Could you check a few things on this model? Use its own coordinates, in mm. Give positions to 0.01 mm unless a question says otherwise; leave off trailing zeros. Loops run counter-clockwise (first coordinate to the right, second up) from the corner with the lowest first, then second, coordinate; pieces in that order, holes last. Notation, with made-up numbers: (-28, -38) - (-15, -38) arc R28 cw to (-15, -1) - close; hole circle Ø3 at (-38, -2.5). An arc over 180 degrees is marked (long way). Write each question's results on one line, items separated by ' | '. Start each with the question number.
1) I want a section at C-C, the plane z = -159.5. Write out the boundary of the cut face in (x, y) (3 decimals).
2) I want a section at A-A, the plane y = -56. Write out the boundary of the cut face in (x, z).
3) If I drill on probe 1 along Z at (x, y) = (187, 12) (3 decimals); probe 2 along Z at (x, y) = (210, -17) (3 decimals); probe 3 along Y at (x, z) = (238, -112), over which ranges is the centre line in solid material (lowest first)? Write a range as [from, to].
4) I'm going to push flat-ended pins straight in: pin 1 (8 mm diameter, centred on x = 149.5, y = -143, fed in from -Z); pin 2 (15 mm diameter, centred on x = -2.5, z = 34.5, fed in from +Y); pin 3 (8 mm diameter, centred on x = 209.5, y = -24, fed in from +Z) (3 decimals). Where does each tip first touch, or does it pass through?
5) I want a section at B-B, the plane y = 7.5. Write out the boundary of the cut face in (x, z) (3 decimals).
6) I want a section at D-D, the plane x = 194. Count the separate pieces of the cut face and the enclosed holes in it, and give its area (3 significant figures).
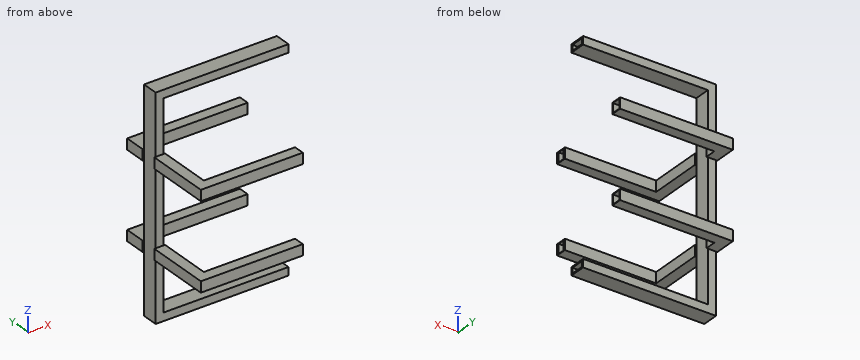
Autodesk Inventor part; units mm, degrees
ref_plane "Work Plane2" through (304.8, 0, 0) normal (1, 0, 0) x (0, 1, 0)
ref_plane "Work Plane3" through (0, 0, 38.1) normal (0, 0, 1) x (1, 0, 0)
ref_plane "Work Plane5" through (0, 0, 101.6) normal (0, 0, 1) x (1, 0, 0)
sketch "Sketch10" plane through (0, 0, 0) normal (0, 1, 0) x (-1, 0, 0)
  line L0 (0, 0) -> (0, 247.65)
  line L1 (0, 247.65) -> (-304.8, 247.65)
  line L2 (0, 0) -> (-304.8, 0) construction
  line L3 (0, 0) -> (0, -247.65)
  line L4 (0, -247.65) -> (-304.8, -247.65)
  dimension "d31" = 247.65
  dimension "d32" = 304.8
ref_plane "Work Plane2" through (304.8, 0, 0) normal (1, 0, 0) x (0, 1, 0)
sketch "Sketch11" plane through (304.8, 0, 0) normal (1, 0, 0) x (0, 1, 0)
  line L0 (-19.05, 257.175) -> (-19.05, 238.125)
  line L1 (-19.05, 238.125) -> (19.05, 238.125)
  line L2 (19.05, 238.125) -> (19.05, 257.175)
  line L3 (19.05, 257.175) -> (-19.05, 257.175)
  line L4 (-19.05, 257.175) -> (19.05, 238.125) construction
  line L5 (-19.05, 238.125) -> (19.05, 257.175) construction
  line L6 (-15.875, 254) -> (-15.875, 241.3)
  line L7 (-15.875, 241.3) -> (15.875, 241.3)
  line L8 (15.875, 241.3) -> (15.875, 254)
  line L9 (15.875, 254) -> (-15.875, 254)
  line L10 (-15.875, 254) -> (15.875, 241.3) construction
  line L11 (-15.875, 241.3) -> (15.875, 254) construction
  point P0 (0, 0)
  point P1 (0, 247.65)
  dimension "d34" = 247.65
  dimension "d35" = 19.05
  dimension "d36" = 38.1
  dimension "d37" = 3.175
  dimension "d38" = 3.175
sweep "Sweep5" add profiles "Sketch11" path "Sketch10"
sketch "Sketch12" plane through (304.8, 19.05, 257.175) normal (0, 1, 0) x (1, 0, 0)
  line L0 (-304.8, 257.175) -> (-304.8, 0) construction
  line L1 (0, 0) -> (-314.325, 0) construction
  line L2 (-317.5, 142.875) -> (-292.1, 142.875)
  line L3 (-292.1, 142.875) -> (-292.1, 168.275)
  line L4 (-292.1, 168.275) -> (-317.5, 168.275)
  line L5 (-317.5, 168.275) -> (-317.5, 142.875)
  line L6 (-317.5, 142.875) -> (-292.1, 168.275) construction
  line L7 (-292.1, 142.875) -> (-317.5, 168.275) construction
  line L8 (-298.45, 15.875) -> (-298.45, 498.475)
  line L9 (-315.9125, 144.4625) -> (-293.6875, 144.4625)
  line L10 (-293.6875, 144.4625) -> (-293.6875, 166.6875)
  line L11 (-293.6875, 166.6875) -> (-315.9125, 166.6875)
  line L12 (-315.9125, 166.6875) -> (-315.9125, 144.4625)
  line L13 (-315.9125, 144.4625) -> (-293.6875, 166.6875) construction
  line L14 (-293.6875, 144.4625) -> (-315.9125, 166.6875) construction
  point P0 (-304.8, 155.575)
  dimension "d41" = 25.4
  dimension "d42" = 25.4
  dimension "d43" = 101.6
  dimension "d44" = 1.5875
  dimension "d45" = 1.5875
ref_plane "Work Plane3" through (0, 0, 38.1) normal (0, 0, 1) x (1, 0, 0)
sketch "Sketch13" plane through (0, 0, 38.1) normal (0, 0, 1) x (1, 0, 0)
  line L0 (304.8, 19.05) -> (-9.525, 19.05)
  line L1 (0, 19.05) -> (0, 57.15)
  line L2 (0, 57.15) -> (254, 57.15)
  point P0 (0, 0)
  dimension "d47" = 254
  dimension "d48" = 38.1
sweep "Sweep6" add profiles "Sketch12" path "Sketch13" path curves L1 L2 contours L5 L4 L8 L11 L12 L9 L2 | L8 L9 L10 L11 L4 L3 L2
mirror "Mirror2" about plane through (0, 0, 0) normal (0, 0, 1) of "Sweep6"
sketch "Sketch14" plane through (304.8, -19.05, 238.125) normal (0, -1, 0) x (1, 0, 0)
  line L0 (-304.8, -238.125) -> (-304.8, 15.875) construction
  line L1 (0, 15.875) -> (-311.15, 15.875) construction
  line L2 (-317.5, -123.825) -> (-317.5, -149.225)
  line L3 (-317.5, -149.225) -> (-292.1, -149.225)
  line L4 (-292.1, -149.225) -> (-292.1, -123.825)
  line L5 (-292.1, -123.825) -> (-317.5, -123.825)
  line L6 (-317.5, -123.825) -> (-292.1, -149.225) construction
  line L7 (-317.5, -149.225) -> (-292.1, -123.825) construction
  line L8 (-312.7375, -125.4125) -> (-312.7375, -147.6375)
  line L9 (-312.7375, -147.6375) -> (-296.8625, -147.6375)
  line L10 (-296.8625, -147.6375) -> (-296.8625, -125.4125)
  line L11 (-296.8625, -125.4125) -> (-312.7375, -125.4125)
  line L12 (-312.7375, -125.4125) -> (-296.8625, -147.6375) construction
  line L13 (-312.7375, -147.6375) -> (-296.8625, -125.4125) construction
  line L14 (-314.325, 19.05) -> (-314.325, -495.3)
  point P0 (-304.8, -136.525)
  dimension "d52" = 101.6
  dimension "d53" = 25.4
  dimension "d54" = 25.4
  dimension "d55" = 1.5875
  dimension "d56" = 1.5875
ref_plane "Work Plane5" through (0, 0, 101.6) normal (0, 0, 1) x (1, 0, 0)
sketch "Sketch15" plane through (0, 0, 101.6) normal (0, 0, 1) x (1, 0, 0)
  line L0 (-9.525, -19.05) -> (304.8, -19.05)
  line L1 (0, -19.05) -> (0, -158.75)
  line L2 (0, -158.75) -> (228.6, -158.75)
  point P0 (0, 0)
  dimension "d58" = 228.6
  dimension "d59" = 139.7
sweep "Sweep7" add profiles "Sketch14" path "Sketch15" path curves L1 L2
mirror "Mirror5" about plane through (0, 0, 0) normal (0, 0, 1) of "Sweep7"
ref_plane "Work Plane6" through (152.4, 0, 0) normal (1, 0, 0) x (0, 1, 0)
equation "\"d31\" = halfOfWidth"
equation "\"d32\" = length"
equation "\"d35\" = largeTubingWidth"
equation "\"d36\" = largeTubingHeight"
equation "\"d37\" = largeTubeThickness"
equation "\"d38\" = largeTubeThickness"
equation "\"d41\" = smallSupportTubeWidth"
equation "\"d42\" = smallSupportTubeWidth"
equation "\"d44\" = smallSupportTubeThickness"
equation "\"d45\" = smallSupportTubeThickness"
equation "\"d47\" = topSupportTubeExtension"
equation "\"d48\" = smallSupportTubeLength"
equation "\"d53\" = smallSupportTubeWidth"
equation "\"d54\" = smallSupportTubeHeight"
equation "\"d55\" = smallSupportTubeThickness"
equation "\"d56\" = smallSupportTubeThickness"
equation "\"d58\" = bottomSupportTubeExtension"
equation "\"halfOfWidth\" = 0.5 * width"
equation "\"length\" = 304.8"
equation "\"height\" = 241.3"
equation "\"largeTubingWidth\" = 19.05"
equation "\"largeTubingHeight\" = 38.1"
equation "\"largeTubeThickness\" = 3.175"
equation "\"d33\" = length"
equation "\"width\" = 495.3"
equation "\"smallSupportTubeWidth\" = 25.4"
equation "\"smallSupportTubeHeight\" = 25.4"
equation "\"smallSupportTubeThickness\" = 1.5875"
equation "\"distaceToMiddleSmallSupportTube\" = 101.6"
equation "\"smallSupportTubeLength\" = 38.1"
equation "\"d46\" = smallSupportTubeLength"
equation "\"d57\" = distaceToMiddleSmallSupportTube"
equation "\"distanceOriginToPlaneForSupportTubes\" = 152.4"
equation "\"d62\" = distanceOriginToPlaneForSupportTubes"
properties part number "ShooterFrame"
Answers:
1) outline: (-9.525, -19.05) - (9.525, -19.05) - (9.525, 19.05) - (-9.525, 19.05) - close; hole (-6.35, -15.875) - (6.35, -15.875) - (6.35, 15.875) - (-6.35, 15.875) - close
2) outline: (-12.7, -114.3) - (12.7, -114.3) - (12.7, -88.9) - (-12.7, -88.9) - close; (-12.7, 88.9) - (12.7, 88.9) - (12.7, 114.3) - (-12.7, 114.3) - close; hole (-7.94, -112.71) - (7.94, -112.71) - (7.94, -90.49) - (-7.94, -90.49) - close; hole (-7.94, 90.49) - (7.94, 90.49) - (7.94, 112.71) - (-7.94, 112.71) - close
3) probe 1: z = [-257.175, -254], [-241.3, -238.125], [238.125, 241.3], [254, 257.175] | probe 2: z = [-257.175, -238.125], [238.125, 257.175] | probe 3: y = [44.45, 46.04], [68.26, 69.85]
4) pin 1: stops at z = -114.3 | pin 2: stops at y = 19.05 | pin 3: passes through
5) outline: (-9.525, -257.175) - (304.8, -257.175) - (304.8, -254) - (-6.35, -254) - (-6.35, 254) - (304.8, 254) - (304.8, 257.175) - (-9.525, 257.175) - close; (6.35, -241.3) - (304.8, -241.3) - (304.8, -238.125) - (9.525, -238.125) - (9.525, 238.125) - (304.8, 238.125) - (304.8, 241.3) - (6.35, 241.3) - close
6) separate pieces: 6 | enclosed holes: 6 | area: 1,530 mm2
